Read the model definition and answer for the solid it produces. Units are mm, in the model's axes. A direction names the side the tool comes from. Give positions to 0.01 mm unless a question says otherwise; leave off trailing zeros. Loops run counter-clockwise (first coordinate to the right, second up) from the corner with the lowest first, then second, coordinate; pieces in that order, holes last.
(1) Which of the six approach directions +Z, -Z, +X, -X, +Y, -Y give full straight-line access (tool end or side, diameter ignored) to faces 1 (the face through (-70, 0, 2)), 2 (the face through (0, 95, 2)), 3 (the face through (72, -20, 2))?
(2) Each of these flat-tipped pins is pushed along its axis until it touches: P1, Ø1, axis at x = -10.5, z = 1.5, coming from the -Y side; P2, Ø4.5, axis at x = 38.18, y = -38.18, coming from the +Z side; P3, Ø3.5, axis at x = 38.18, y = 38.18, coming from the -Z side. Where does it stop, or does it pass through?
(3) Find section A-A, the plane y = 0. Write down the section's boundary in (x, z), then the cut area to 3 significant figures.
(4) Find section C-C, the plane z = 0.85. Write down the section's boundary in (x, y).
(5) Straight lines are drawn through the part: probe 1 along Y at (x, z) = (0, 1.1); probe 2 along X at (y, z) = (0, 2.1); probe 3 along Z at (x, y) = (-52, -22.5). For each, find the intervals that lie inside material, in ascending order.
(6) Find section B-B, the plane x = -2.5. Write down the section's boundary in (y, z).
(7) Determine the mould class of faces 4 (the face through (72, 20, 2)), 5 (the face through (75, 59, 2)), 6 (the face through (37.75, -40.136, 1.479)), 7 (the face through (36.186, 38.272, 1.479)) for opening direction X: pulls with the +X half, pulls with the -X half, needs draft (parallel to the pull), parting line crosses it, or undercut.
```python
from build123d import *

# Parameters (mm, degrees)
CROQUIS1_W              = 150
CROQUIS1_H              = 200
CROQUIS1_R              = 46.5
CROQUIS1_R_2            = 2
SALIENTE_EXTRUIR1_DEPTH = 5
CROQUIS2_R              = 58
CORTAR_EXTRUIR1_DEPTH   = 2
CORTAR_EXTRUIR2_START   = -5
CROQUIS3_W              = 40
CROQUIS3_H              = 5
CROQUIS3_W_2            = 5
CROQUIS3_H_2            = 40
CORTAR_EXTRUIR2_DEPTH   = 5


with BuildPart() as part:
    # Croquis1 → Saliente-Extruir1 (new body)
    with BuildSketch(Plane.XY):
        Rectangle(CROQUIS1_W, CROQUIS1_H)
        Circle(CROQUIS1_R, mode=Mode.SUBTRACT)
        with Locations((-38.183766184, 38.183766184)):
            Circle(CROQUIS1_R_2, mode=Mode.SUBTRACT)
        with Locations((38.183766184, 38.183766184)):
            Circle(CROQUIS1_R_2, mode=Mode.SUBTRACT)
        with Locations((38.183766184, -38.183766184)):
            Circle(CROQUIS1_R_2, mode=Mode.SUBTRACT)
        with Locations((-38.183766184, -38.183766184)):
            Circle(CROQUIS1_R_2, mode=Mode.SUBTRACT)
    extrude(amount=SALIENTE_EXTRUIR1_DEPTH)

    # Croquis2 → Cortar-Extruir1 (cut)
    with BuildSketch(Plane.XY.offset(5)):
        Circle(CROQUIS2_R)
    extrude(amount=-CORTAR_EXTRUIR1_DEPTH, mode=Mode.SUBTRACT)

    # Croquis3 → Cortar-Extruir2 (cut)
    with BuildSketch(Plane.XY.offset(5).offset(CORTAR_EXTRUIR2_START)):
        with Locations((0, 97.5)):
            Rectangle(CROQUIS3_W, CROQUIS3_H)
        with Locations((0, -97.5)):
            Rectangle(CROQUIS3_W, CROQUIS3_H)
        with Locations((-72.5, 0)):
            Rectangle(CROQUIS3_W_2, CROQUIS3_H_2)
        with Locations((72.5, 0)):
            Rectangle(CROQUIS3_W_2, CROQUIS3_H_2)
    extrude(amount=CORTAR_EXTRUIR2_DEPTH, mode=Mode.SUBTRACT)


solid = part.part
```
Entries:
1. face 1: +Z, -Z, -X
1. face 2: +Z, -Z, +Y
1. face 3: +Z, -Z, +X
2. P1: stops at y = -95
2. P2: stops at z = 3
2. P3: passes through
3. outline: (-70, 0) - (-46.5, 0) - (-46.5, 3) - (-58, 3) - (-58, 5) - (-70, 5) - close; (46.5, 0) - (70, 0) - (70, 5) - (58, 5) - (58, 3) - (46.5, 3) - close
3. area: 189 mm2
4. outline: (-75, -100) - (-20, -100) - (-20, -95) - (20, -95) - (20, -100) - (75, -100) - (75, -20) - (70, -20) - (70, 20) - (75, 20) - (75, 100) - (20, 100) - (20, 95) - (-20, 95) - (-20, 100) - (-75, 100) - (-75, 20) - (-70, 20) - (-70, -20) - (-75, -20) - close; hole circle Ø93 at (0, 0); hole circle Ø4 at (-38.18, -38.18); hole circle Ø4 at (-38.18, 38.18); hole circle Ø4 at (38.18, -38.18); hole circle Ø4 at (38.18, 38.18)
5. probe 1: y = -95 to -46.5, 46.5 to 95
5. probe 2: x = -70 to -46.5, 46.5 to 70
5. probe 3: z = 0 to 3
6. outline: (-95, 0) - (-46.43, 0) - (-46.43, 3) - (-57.95, 3) - (-57.95, 5) - (-95, 5) - close; (46.43, 0) - (95, 0) - (95, 5) - (57.95, 5) - (57.95, 3) - (46.43, 3) - close
7. face 4: needs draft
7. face 5: pulls with the +X half
7. face 6: undercut
7. face 7: undercut
